Autodesk Fusion 360 part; units mm, degrees
sketch "Sketch1" plane through (0, 0, 0) normal (0, 1, 0) x (1, 0, 0)
  line L0 (0, 0) -> (-15, 0)
  line L1 (-15, 0) -> (-15, -6)
  line L2 (-15, -6) -> (-20, -6)
  line L3 (-20, -6) -> (-20, 0)
  line L4 (-20, 0) -> (-25, 0)
  line L5 (-7.5, 20) -> (0, 20)
  line L6 (0, 0) -> (15, 0)
  line L7 (15, 0) -> (15, -6)
  line L8 (15, -6) -> (20, -6)
  line L9 (20, -6) -> (20, 0)
  line L10 (20, 0) -> (25, 0)
  line L11 (7.5, 20) -> (0, 20)
  line L12 (-25, 0) -> (-11.5, 18)
  line L13 (25, 0) -> (11.5, 18)
  arc A0 (-7.5, 20) -> (-11.5, 18) centre (-7.5, 15) ccw
  arc A1 (11.5, 18) -> (7.5, 20) centre (7.5, 15) ccw
  line L14 (0, 13) -> (-4.5, 13)
  line L15 (-4.5, 13) -> (-4.5, 7.5)
  line L16 (-4.5, 7.5) -> (4.5, 7.5)
  line L17 (0, 13) -> (4.5, 13)
  line L18 (4.5, 13) -> (4.5, 7.5)
  circle A2 centre (0, 2.5) radius 1.5
  dimension "d1" = 5
  dimension "d6" = 2.5
  dimension "d7" = 3
extrude "Extrude1" add sketch "Sketch1" along normal blind 5
Here's how the part is built. I have some questions about the finished solid (model axes, mm). A direction names the side the tool comes from. Give positions to 0.01 mm unless a question says otherwise; leave off trailing zeros. Write each loop counter-clockwise with the first axis right and the second up, starting at its lowest first coordinate (ties: lowest second). Pieces come first, ordered by that corner, then holes. Notation, with made-up numbers: (13, -15) -> (33, -15) arc R26 cw to (33, 24) -> close; hole circle Ø9 at (-0.75, 89). An arc over 180 degrees is marked (long way). Use one line per item in the form item = value. Start each with the question number.
1. Thinking about a two-plate mould opening in Z: for faces 5 (the face through (0, 2, -13)), 6 (the face through (18.344, 2.465, -8.874)), 7 (the face through (0, 0, -7)), which applies, +Z half, -Z half, draft (parallel to the pull), parting line (faces both ways), or undercut?
2. Imagine slicing it at A-A on x = 0. List the corners of the cut face in (y, z) for me, plus the area to 3 significant figures.
3. On a 3-axis mill with a long thin cutter (end or side, diameter ignored), from which of +Z, -Z, +X, -X, +Y, -Y can I reach the whole of each face in a straight line? I mean faces 1 (the face through (-4.5, 2, -10)), 2 (the face through (-15, 2, 3)), 3 (the face through (-22, 2, 0)), 4 (the face through (20, 2, 3)). Say none if no direction works.
4. Imagine slicing it at B-B on y = 3.3. List the corners of the cut face in (x, z) for me, plus the area to 3 significant figures.
5. Will these pins go through, and if not, where does the flat tip stop? pin 1 Ø2.5 at (y, z) = (3, 3.5) entering from -X; pin 2 Ø2.5 at (x, y) = (0, 2) entering from +Z.
6. Imagine slicing it at C-C on z = 2.75. List the corners of the cut face in (x, y) for me.
7. Imagine slicing it at D-D on z = -17. List the corners of the cut face in (x, y) for me, plus the area to 4 significant figures.
8. If I drill on L1, parallel to Z at x = 0, y = 2.75; L2, parallel to X at y = 2.45, z = 1.75; L3, parallel to X at y = 3.6, z = -9.5 (3 decimals), over which ranges is the centre line in solid material (lowest first)?
Entries:
q1.face_5 = undercut
q1.face_6 = -Z half
q1.face_7 = draft
q2.outline = (0, -20) -> (5, -20) -> (5, -13) -> (0, -13) -> close; (0, -7.5) -> (5, -7.5) -> (5, -4) -> (0, -4) -> close; (0, -1) -> (5, -1) -> (5, 0) -> (0, 0) -> close
q2.area = 57.5 mm²
q3.face_1 = +Y, -Y
q3.face_2 = +Z, +Y, -Y
q3.face_3 = +Z, -X, +Y, -Y
q3.face_4 = +Z, +X, +Y, -Y
q4.outline = (-25, 0) -> (-11.5, -18) arc R5 ccw to (-7.5, -20) -> (7.5, -20) arc R5 ccw to (11.5, -18) -> (25, 0) -> (20, 0) -> (20, 6) -> (15, 6) -> (15, 0) -> (-15, 0) -> (-15, 6) -> (-20, 6) -> (-20, 0) -> close; hole (-4.5, -13) -> (4.5, -13) -> (4.5, -7.5) -> (-4.5, -7.5) -> close; hole circle Ø3 at (0, -2.5)
q4.area = 702 mm²
q5.pin_1 = -20
q5.pin_2 = 0
q6.outline = (-20, 0) -> (-15, 0) -> (-15, 5) -> (-20, 5) -> close; (15, 0) -> (20, 0) -> (20, 5) -> (15, 5) -> close
q7.outline = (-12.25, 0) -> (12.25, 0) -> (12.25, 5) -> (-12.25, 5) -> close
q7.area = 122.5 mm²
q8.L1 = -20 to -13, -7.5 to -4, -1 to 0
q8.L2 = -20 to -15, 15 to 20
q8.L3 = -17.875 to -4.5, 4.5 to 17.875
